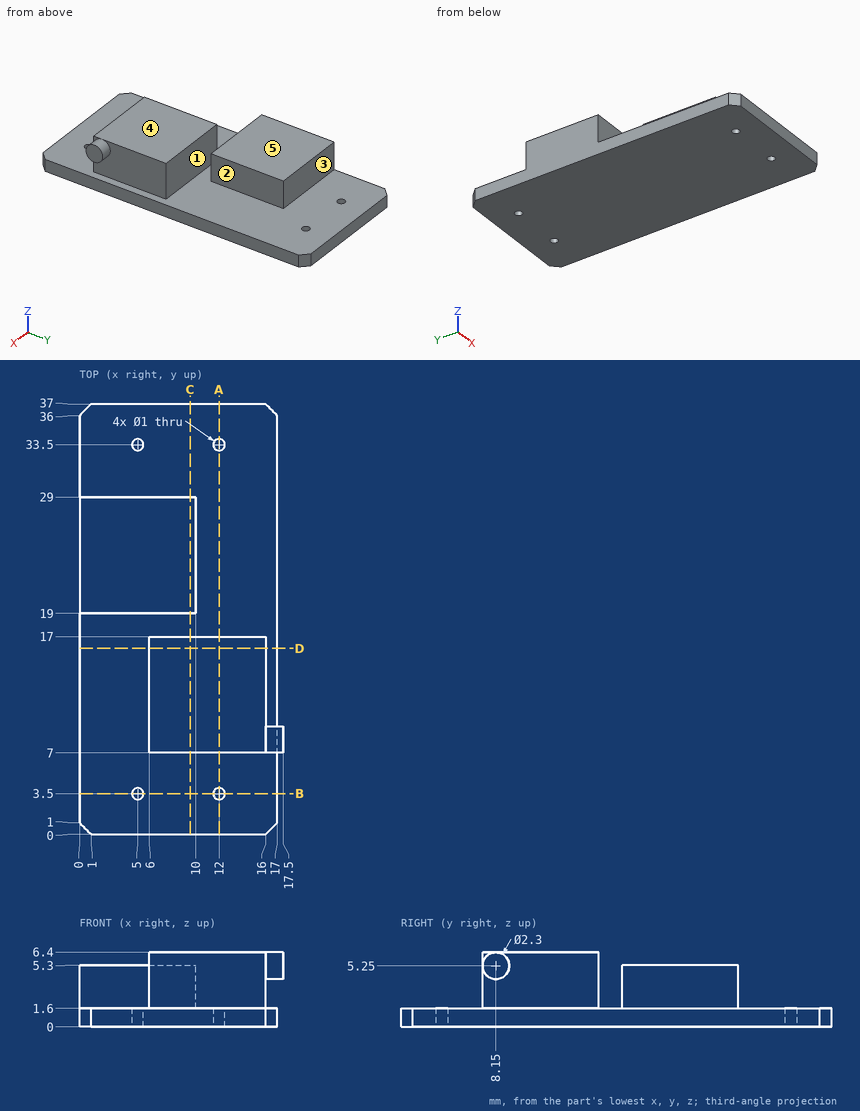
Can you work these out from the drawing? Everything is in mm from the part's minimum corner. A direction names the side the tool comes from. Coordinates: 2 decimals unless noted, no trailing zeros. Write each loop counter-clockwise with the first axis right and the second up, starting at its lowest first coordinate (ties: lowest second). Pieces come first, ordered by that corner, then holes. Notation, with made-up numbers: (50.25, 79) -> (109.25, 79) arc R25 cw to (109.25, 118) -> close; hole circle Ø6 at (43.25, 87.5). An arc over 180 degrees is marked (long way). Return JSON: item names as keys, results as strings.
(1) We'd pull the mould along Y, two halves only. Please class the marked faces 1, 2 and 3: +Y half, -Y half, draft (parallel to the pull), parting line (faces both ways), or undercut.
Numbers:
{"face 1": "undercut", "face 2": "draft", "face 3": "+Y half"}
(2) I'm going to push flat-ended pins straight in: pin 1 (1.8 mm diameter, centred on x = 5, z = 3.5, fed in from +Y); pin 2 (1 mm diameter, centred on x = 15.5, z = 5.5, fed in from -Y); pin 3 (2.5 mm diameter, centred on y = 12, z = 4, fed in from +X); pin 4 (3 mm diameter, centred on x = 5.5, z = 3, fed in from -Y). Where does each tip first touch, or does it pass through?
Numbers:
{"pin 1": "stops at y = 29", "pin 2": "stops at y = 7", "pin 3": "stops at x = 16", "pin 4": "stops at y = 0"}
(3) Imagine slicing it at C-C, the plane x = 9.5. Please give me the cut outline in (y, z), then the cut area to 3 significant figures.
Numbers:
{"outline": "(0, 0) -> (37, 0) -> (37, 1.6) -> (29, 1.6) -> (29, 5.3) -> (19, 5.3) -> (19, 1.6) -> (17, 1.6) -> (17, 6.4) -> (7, 6.4) -> (7, 1.6) -> (0, 1.6) -> close", "area": "144 mm2"}
(4) Which directions (+Z, -Z, +X, -X, +Y, -Y) give clear straight access to the entire face, cutting with the end or side of a thin tool? Please do the marked faces 4 and 5.
Numbers:
{"face 4": "+Z, +X, -X, +Y, -Y", "face 5": "+Z, +X, -X, +Y"}
(5) Imagine slicing it at B-B, the plane y = 3.5. Please give me the cut outline in (x, z), then the cut area to 3 significant figures.
Numbers:
{"outline": "(0, 0) -> (4.5, 0) -> (4.5, 1.6) -> (0, 1.6) -> close; (5.5, 0) -> (11.5, 0) -> (11.5, 1.6) -> (5.5, 1.6) -> close; (12.5, 0) -> (17, 0) -> (17, 1.6) -> (12.5, 1.6) -> close", "area": "24.0 mm2"}
(6) I need wall thicknesses on L1, parallel to Y at x = 12, z = 0.65; L2, parallel to X at y = 33.5, z = 0.9; L3, parallel to Y at x = 6.5, z = 4.75. Which ranges of each line are inside material? Lowest first, please.
Numbers:
{"L1": "y = 0 to 3, 4 to 33, 34 to 37", "L2": "x = 0 to 4.5, 5.5 to 11.5, 12.5 to 17", "L3": "y = 7 to 17, 19 to 29"}
(7) Imagine slicing it at A-A, the plane x = 12. Please give me the cut outline in (y, z).
Numbers:
{"outline": "(0, 0) -> (3, 0) -> (3, 1.6) -> (0, 1.6) -> close; (4, 0) -> (33, 0) -> (33, 1.6) -> (17, 1.6) -> (17, 6.4) -> (7, 6.4) -> (7, 1.6) -> (4, 1.6) -> close; (34, 0) -> (37, 0) -> (37, 1.6) -> (34, 1.6) -> close"}
(8) Imagine slicing it at D-D, the plane y = 16. Please give me the cut outline in (x, z).
Numbers:
{"outline": "(0, 0) -> (17, 0) -> (17, 1.6) -> (16, 1.6) -> (16, 6.4) -> (6, 6.4) -> (6, 1.6) -> (0, 1.6) -> close"}
